```python
from build123d import *

# Parameters (mm, degrees)
SKETCH1_R           = 1.5
BOSS_EXTRUDE3_DEPTH = 4
SKETCH2_W           = 4
SKETCH2_H           = 61.93693974
BOSS_EXTRUDE4_DEPTH = 60
SKETCH3_R           = 1.5
CUT_EXTRUDE2_DEPTH  = 10


with BuildPart() as part:
    # Sketch1 → Boss-Extrude3 (new body)
    with BuildSketch(Plane.XY):
        with BuildLine():
            Line((0, 61.171572875), (0, 0))
            Line((0, 0), (51, 0))
            Line((51, 0), (51, 61.171572875))
            ThreePointArc((51, 61.171572875), (50.847759065, 61.93693974), (50.414213562, 62.585786438))
            Line((50.414213562, 62.585786438), (46.585786438, 66.414213562))
            ThreePointArc((46.585786438, 66.414213562), (45.93693974, 66.847759065), (45.171572875, 67))
            Line((45.171572875, 67), (5.828427125, 67))
            ThreePointArc((5.828427125, 67), (5.06306026, 66.847759065), (4.414213562, 66.414213562))
            Line((4.414213562, 66.414213562), (0.585786438, 62.585786438))
            ThreePointArc((0.585786438, 62.585786438), (0.152240935, 61.93693974), (0, 61.171572875))
        make_face()
        with Locations((19.55, 11.7)):
            Circle(SKETCH1_R, mode=Mode.SUBTRACT)
        with Locations((31.45, 11.7)):
            Circle(SKETCH1_R, mode=Mode.SUBTRACT)
        with Locations((31.45, 60.8)):
            Circle(SKETCH1_R, mode=Mode.SUBTRACT)
        with Locations((19.55, 60.8)):
            Circle(SKETCH1_R, mode=Mode.SUBTRACT)
        with BuildLine():
            Line((15.25, 56.5), (35.75, 56.5))
            Line((35.75, 56.5), (35.75, 35.324710973))
            ThreePointArc((35.75, 35.324710973), (36.625, 31), (35.75, 26.675289027))
            Line((35.75, 26.675289027), (35.75, 16))
            Line((35.75, 16), (15.25, 16))
            Line((15.25, 16), (15.25, 26.675289027))
            ThreePointArc((15.25, 26.675289027), (14.375, 31), (15.25, 35.324710973))
            Line((15.25, 35.324710973), (15.25, 56.5))
        make_face(mode=Mode.SUBTRACT)
    extrude(amount=BOSS_EXTRUDE3_DEPTH)

    # Sketch2 → Boss-Extrude4 (add)
    with BuildSketch(Plane(origin=(0, 0, 0), x_dir=(-1, 0, 0), z_dir=(0, 0, -1))):
        with Locations((-2.152240935, 30.96846987)):
            Rectangle(SKETCH2_W, SKETCH2_H)
    extrude(amount=BOSS_EXTRUDE4_DEPTH)

    # Sketch3 → Cut-Extrude2 (cut)
    with BuildSketch(Plane.ZY.offset(-0.152240935)):
        with Locations((-46, 30.96846987)):
            Circle(SKETCH3_R)
        with Locations((-36, 30.96846987)):
            Circle(SKETCH3_R)
    extrude(amount=-CUT_EXTRUDE2_DEPTH, mode=Mode.SUBTRACT)


solid = part.part
```
Check sheet for the modelled part. Datum: model origin and axes. Units: mm. A direction names the side the tool comes from. Give positions to 0.01 mm unless a question says otherwise; leave off trailing zeros. Loops run counter-clockwise (first coordinate to the right, second up) from the corner with the lowest first, then second, coordinate; pieces in that order, holes last. Notation, with made-up numbers: M -19,44.5 L -4,44.5 A22 cw -4,57.5 Z; hole C -31.5,-8.5 d2. An arc over 180 degrees is marked long. Answer in a Markdown table with one row per item.
1) Cross-section at D-D (y = 42.5). Enter the section's corners in (x, z), plus the area to 3 significant figures.
Solutions:
| item | result |
|---|---|
| outline | M 0,0 L 0.15,0 L 0.15,-60 L 4.15,-60 L 4.15,0 L 15.25,0 L 15.25,4 L 0,4 Z; M 35.75,0 L 51,0 L 51,4 L 35.75,4 Z |
| area | 362 mm^2 |
2) Tool access check on faces 5 (the face through (51, 30, 2)), 6 (the face through (0.152, 31, -30)), 7 (the face through (35.75, 21, 2)), 8 (the face through (2, 61.937, -30)). Record the directions out of +Z, -Z, +X, -X, +Y, -Y that give a thin tool (end or side, any length) a straight path to the whole face; none if there is none.
Solutions:
| item | result |
|---|---|
| face 5 | +Z, -Z, +X, +Y, -Y |
| face 6 | -Z, -X, +Y, -Y |
| face 7 | +Z, -Z |
| face 8 | -Z, +X, -X, +Y |
3) Cross-section at B-B (y = 11.7). Enter the section's corners in (x, z).
Solutions:
| item | result |
|---|---|
| outline | M 0,0 L 0.15,0 L 0.15,-60 L 4.15,-60 L 4.15,0 L 18.05,0 L 18.05,4 L 0,4 Z; M 21.05,0 L 29.95,0 L 29.95,4 L 21.05,4 Z; M 32.95,0 L 51,0 L 51,4 L 32.95,4 Z |
4) Depth check by flat-ended pin: pin 1 (12 mm diameter, centred on y = 11, z = -28.5, fed in from +X); pin 2 (1.5 mm diameter, centred on x = 38.5, y = 23.5, fed in from -Z); pin 3 (1.2 mm diameter, centred on x = 2, z = -23, fed in from +Y). Enter the tip coordinate at first touch or a pass-through.
Solutions:
| item | result |
|---|---|
| pin 1 | stops at x = 4.15 |
| pin 2 | stops at z = 0 |
| pin 3 | stops at y = 61.94 |
5) Thickness scan on line 1 (Y direction, x = 31.45, z = 2.15); line 2 (Y direction, x = 2.5, z = -46); line 3 (Z direction, x = 25, y = 6). Record the ranges inside material, lowest first.
Solutions:
| item | result |
|---|---|
| line 1 | y = 0 to 10.2, 13.2 to 16, 56.5 to 59.3, 62.3 to 67 |
| line 2 | y = 0 to 29.47, 32.47 to 61.94 |
| line 3 | z = 0 to 4 |
6) Cross-section at A-A (x = 31.45). Enter the section's corners in (y, z), plus the area to 3 significant figures.
Solutions:
| item | result |
|---|---|
| outline | M 0,0 L 10.2,0 L 10.2,4 L 0,4 Z; M 13.2,0 L 16,0 L 16,4 L 13.2,4 Z; M 56.5,0 L 59.3,0 L 59.3,4 L 56.5,4 Z; M 62.3,0 L 67,0 L 67,4 L 62.3,4 Z |
| area | 82.0 mm^2 |
7) Mould release check, pull along Y, two halves, no side actions. Record for faces 1 (the face through (36.5, 34, 4)), 2 (the face through (2.12, 31.98, -37.11)), 3 (the face through (3, 0, -14)), 4 (the face through (3, 65, 2)): released by +Y, released by -Y, zero draft, split by the parting line, or undercut.
Solutions:
| item | result |
|---|---|
| face 1 | zero draft |
| face 2 | undercut |
| face 3 | released by -Y |
| face 4 | released by +Y |
8) Cross-section at C-C (z = -46). Enter the section's corners in (x, y).
Solutions:
| item | result |
|---|---|
| outline | M 0.15,0 L 4.15,0 L 4.15,29.47 L 0.15,29.47 Z; M 0.15,32.47 L 4.15,32.47 L 4.15,61.94 L 0.15,61.94 Z |
